from build123d import *

# Parameters (mm, degrees)
F0_W     = 365.9882545471
F0_H     = 43.0952832103
F1_DEPTH = 127
F2_R     = 17.6971191765
F2_R_2   = 10.7051972913
F2_R_3   = 13.0240698206
F2_R_4   = 16.9813148573
F2_R_5   = 21.1576979937
F2_R_6   = 15.977077603
F2_R_7   = 52.8296986553
F3_DEPTH = 254
F4_W     = 366.437792778
F4_H     = 113.5783046484
F4_R     = 9.6480808664
F4_R_2   = 10.5544944744
F4_R_3   = 15.7229424231
F4_R_4   = 9.7312286453
F4_R_5   = 11.0489584241
F4_R_6   = 8.9931980907
F4_R_7   = 12.8970231178
F5_DEPTH = 25.4


with BuildPart() as f1:
    # F0 (on Front) → F1 (new body)
    with BuildSketch(Plane.XZ):
        with Locations((-5.7889074087, 69.1454075277)):
            Rectangle(F0_W, F0_H)
    extrude(amount=F1_DEPTH)

    # F2 (on face) → F3 (cut)
    with BuildSketch(Plane.XY.offset(90.6930491328)):
        with Locations((-150.8334428072, -87.9421010613)):
            Circle(F2_R)
        with Locations((-155.9791564941, -23.6207954586)):
            Circle(F2_R_2)
        with Locations((-97.4467620254, -23.6207954586)):
            Circle(F2_R_3)
        with Locations((-75.577519834, -84.7260355949)):
            Circle(F2_R_4)
        with Locations((7.3969732039, -84.082826972)):
            Circle(F2_R_5)
        with Locations((-36.3415181637, -24.2640078068)):
            Circle(F2_R_6)
        with Locations((123.1753155589, -62.2135810554)):
            Circle(F2_R_7)
    extrude(amount=-F3_DEPTH, mode=Mode.SUBTRACT)

    # F4 (on face) → F5 (join)
    with BuildSketch(Plane.XZ.offset(127)):
        with Locations((-5.5641382933, 104.3869182467)):
            Rectangle(F4_W, F4_H)
        with Locations((-150.9379148483, 129.0579885244)):
            Circle(F4_R, mode=Mode.SUBTRACT)
        with Locations((-108.9373454452, 129.0579885244)):
            Circle(F4_R_2, mode=Mode.SUBTRACT)
        with Locations((-53.3483624458, 125.3520548344)):
            Circle(F4_R_3, mode=Mode.SUBTRACT)
        with Locations((0, 125.3520548344)):
            Circle(F4_R_4, mode=Mode.SUBTRACT)
        with Locations((56.5943047404, 125.3520548344)):
            Circle(F4_R_5, mode=Mode.SUBTRACT)
        with Locations((89.9476930499, 127.8226822615)):
            Circle(F4_R_6, mode=Mode.SUBTRACT)
        with Locations((140.5954509974, 125.3520548344)):
            Circle(F4_R_7, mode=Mode.SUBTRACT)
    extrude(amount=F5_DEPTH)


solid = f1.part
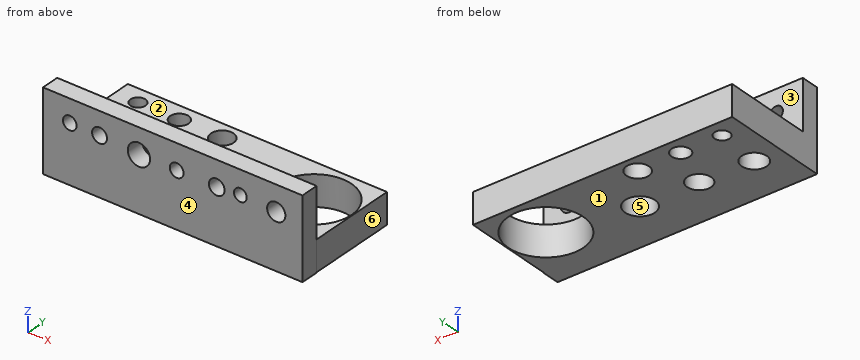
Source: CAD feature listing. Evaluate the final solid. Frame: model axes, mm. Face numbers are marked on the shaded views. A direction names the side the tool comes from. Coordinates: 2 decimals unless noted, no trailing zeros. Loops run counter-clockwise (first coordinate to the right, second up) from the corner with the lowest first, then second, coordinate; pieces in that order, holes last. Notation, with made-up numbers: M 65.5,38.5 L 72.5,38.5 A18 ccw 72.5,72.5 Z; hole C 39.25,36.5 d11. An arc over 180 degrees is marked long. Answer in a Markdown table with one row per item.
Q1. Section D-D on z = 99.5. Return the cut outline in (x, y), plus the area to 3 significant figures.
Answers below:
| item | result |
|---|---|
| outline | M -188.78,-152.4 L 177.65,-152.4 L 177.65,-127 L -188.78,-127 Z |
| area | 9,310 mm^2 |
Q2. First-contact query: pin 1 (22.5 mm diameter, centred on x = 0, z = 125.35, fed in from -Y); pin 2 (1 mm diameter, centred on x = -94, z = 140, fed in from +Y); pin 3 (1.5 mm diameter, centred on x = -146.5, y = -70, fed in from +Z). Flat tips, straight axial feed; report the tip coordinate or a pass-through.
Answers below:
| item | result |
|---|---|
| pin 1 | stops at y = -152.4 |
| pin 2 | stops at y = -127 |
| pin 3 | stops at z = 90.69 |
Q3. Section C-C on y = -53. Return the cut outline in (x, z).
Answers below:
| item | result |
|---|---|
| outline | M -188.78,47.6 L 71.16,47.6 L 71.16,90.69 L -188.78,90.69 Z; M 175.2,47.6 L 177.21,47.6 L 177.21,90.69 L 175.2,90.69 Z |
Q4. Section A-A on z = 63. Return the cut outline in (x, y), plus the area to 3 significant figures.
Answers below:
| item | result |
|---|---|
| outline | M -188.78,-152.4 L 177.65,-152.4 L 177.65,-127 L 177.21,-127 L 177.21,0 L -188.78,0 Z; hole C -150.83,-87.94 d35.39; hole C -155.98,-23.62 d21.41; hole C -97.45,-23.62 d26.05; hole C -75.58,-84.73 d33.96; hole C -36.34,-24.26 d31.95; hole C 7.4,-84.08 d42.32; hole C 123.18,-62.21 d105.66 |
| area | 42,000 mm^2 |
Q5. Set-up query: the marked faces 1 and 2. Return all of +Z, -Z, +X, -X, +Y, -Y with unobstructed straight access to the full face (end or side cutting, diameter ignored); none if empty.
Answers below:
| item | result |
|---|---|
| face 1 | -Z, +X, -X, +Y, -Y |
| face 2 | +Z, +X, -X, +Y |
Q6. Ray query, probe 1 along X at (y, z) = (-96, 55.5); probe 2 along Y at (x, z) = (157.5, 119); probe 3 along Z at (x, y) = (-72, -22). Return the intervals inside material, ascending. Write a range as from..to.
Answers below:
| item | result |
|---|---|
| probe 1 | x = -188.78..-166.59, -135.08..-88.28, -62.88..-10.09, 24.88..82.56, 163.79..177.21 |
| probe 2 | y = -152.4..-127 |
| probe 3 | z = 47.6..90.69 |
Q7. Section B-B on x = 0. Return the cut outline in (y, z).
Answers below:
| item | result |
|---|---|
| outline | M -152.4,47.6 L -103.91,47.6 L -103.91,90.69 L -127,90.69 L -127,115.62 L -152.4,115.62 Z; M -152.4,135.08 L -127,135.08 L -127,161.18 L -152.4,161.18 Z; M -64.26,47.6 L 0,47.6 L 0,90.69 L -64.26,90.69 Z |
Q8. Draft query along Y for the marked faces 3, 4, 5 and 6. Return one class per face: pulls with the +Y half, pulls with the -Y half, needs draft (parallel to the pull), parting line crosses it, or undercut.
Answers below:
| item | result |
|---|---|
| face 3 | pulls with the +Y half |
| face 4 | pulls with the -Y half |
| face 5 | undercut |
| face 6 | needs draft |
